Here's how the part is built. I have some questions about the finished solid (model axes, mm). Face numbers are marked on the shaded views. Round coordinates to 2 decimals unless told otherwise and drop trailing zeros. Write each loop counter-clockwise with the first axis right and the second up, starting at its lowest first coordinate (ties: lowest second). Pieces come first, ordered by that corner, then holes. Notation, with made-up numbers: (31.5, 46) - (65.5, 46) arc R24 cw to (65.5, 85) - close; hole circle Ø10 at (-1.5, 35). An arc over 180 degrees is marked (long way). Use one line per item in the form item = value. Start each with the question number.
1. I want a section at B-B, the plane z = 6.25. List the corners of the cut face in (x, y) for me (3 decimals).
2. Will these pins go through, and if not, where does the flat tip stop? pin 1 (2 mm diameter, centred on y = -2.5, z = 7.5, fed in from +X); pin 2 (1.5 mm diameter, centred on y = 3.5, z = 2, fed in from +X); pin 3 (3 mm diameter, centred on x = -0.5, y = 0, fed in from +Z).
3. We'd pull the mould along X, two halves only. Please class the marked faces 1, 2 and 3: +X half, -X half, draft (parallel to the pull), parting line (faces both ways), or undercut.
4. If I drill on line 1 along Y through (x, z) = (0, 5.5) (3 decimals); line 2 along Z through (x, y) = (1, 0.75); line 3 along Z through (x, y) = (3, -3.25) (3 decimals), over which ranges is the centre line in solid material (lowest first)?
Autodesk Inventor part; units mm, degrees
ref_plane "YZ Plane" through (0, 0, 0) normal (1, 0, 0) x (0, 1, 0)
ref_plane "XZ Plane" through (0, 0, 0) normal (0, 1, 0) x (-1, 0, 0)
ref_plane "XY Plane" through (0, 0, 0) normal (0, 0, 1) x (1, 0, 0)
sketch "Sketch1" plane through (0, 0, 0) normal (0, 0, 1) x (1, 0, 0)
  circle A0 centre (0, 0) radius 3.175
  circle A1 centre (0, 0) radius 3.9688
  dimension "d0" = 7.9375
  dimension "d2" = 6.35
extrude "Extrusion1" add sketch "Sketch1" along normal blind 8.7313
sketch "Sketch2" plane through (0, 0, 0) normal (0, 0, -1) x (-1, 0, 0)
  circle A0 centre (0, 0) radius 3.9687
extrude "Extrusion2" add sketch "Sketch2" along normal blind 0.7937
sketch "Sketch3" plane through (0, 0, 8.7313) normal (0, 0, 1) x (1, 0, 0)
  circle A0 centre (0, 0) radius 3.175
  circle A1 centre (0, 0) radius 3.9687
  circle A2 centre (0, 0) radius 4.7625
  dimension "d7" = 9.525
extrude "Extrusion3" add sketch "Sketch3" along normal blind 0.7937 contours A1 | A2
thread "Thread1"
properties part number "threaded_insert_1-4-20"
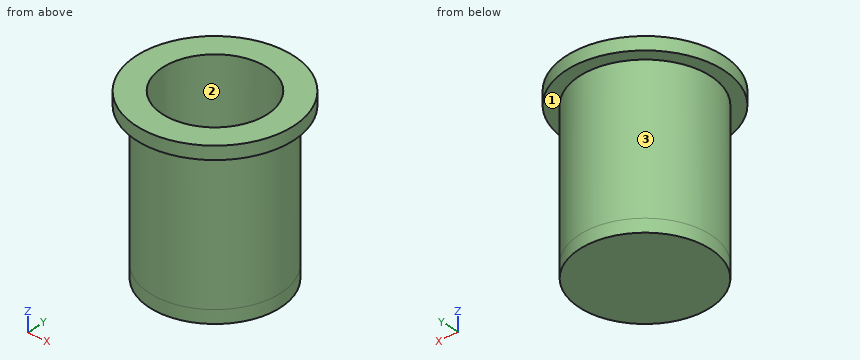
Model answer:
q1.outline = circle Ø7.938 at (0, 0); hole circle Ø6.35 at (0, 0)
q2.pin_1 = 3.67
q2.pin_2 = 2.86
q2.pin_3 = 0
q3.face_1 = draft
q3.face_2 = undercut
q3.face_3 = parting line
q4.line_1 = -3.969 to -3.175, 3.175 to 3.969
q4.line_2 = -0.79 to 0
q4.line_3 = 8.731 to 9.525
